The drawing under review shows one solid part. Ordinate dimensions are in mm from its lowest x, y, z. Coordinates: 2 decimals unless noted, no trailing zeros. Loops run counter-clockwise (first coordinate to the right, second up) from the corner with the lowest first, then second, coordinate; pieces in that order, holes last. Notation, with made-up numbers: M 64.5,25.25 L 96.5,25.25 A8 cw 96.5,31.25 Z; hole C 25.25,12.25 d11. An arc over 180 degrees is marked long. Answer as a JSON object with one key per item and string values. Group by question number.
1. To check wall thickness, follow probe 1 along X at (y, z) = (1.85, 7.25); probe 2 along X at (y, z) = (2.4, 1.25); probe 3 along Z at (x, y) = (25, 0.65). State the ranges of each line that lie inside material, in increasing order.
2. Consider section D-D (x = 13). State the section outline as (y, z) points.
3. Consider section C-C (z = 16.5). State the section outline as (x, y) points, then the cut area to 3 significant figures.
4. Consider section A-A (z = 10.25). State the section outline as (x, y) points, then the cut area to 3 significant figures.
5. Consider section B-B (y = 2.1). State the section outline as (x, z) points, then the cut area to 3 significant figures.
6. Insertion check: pin 1 (1.5 mm diameter, centred on y = 0.5, z = 8, fed in from -X); pin 2 (1.5 mm diameter, centred on y = 2.5, z = 15.5, fed in from +X); pin 3 (1.5 mm diameter, centred on x = 23.5, y = 2, fed in from -Z). Each pin has a flat end and moves straight along its axis. Give the tip position at first contact, or say it passes through.
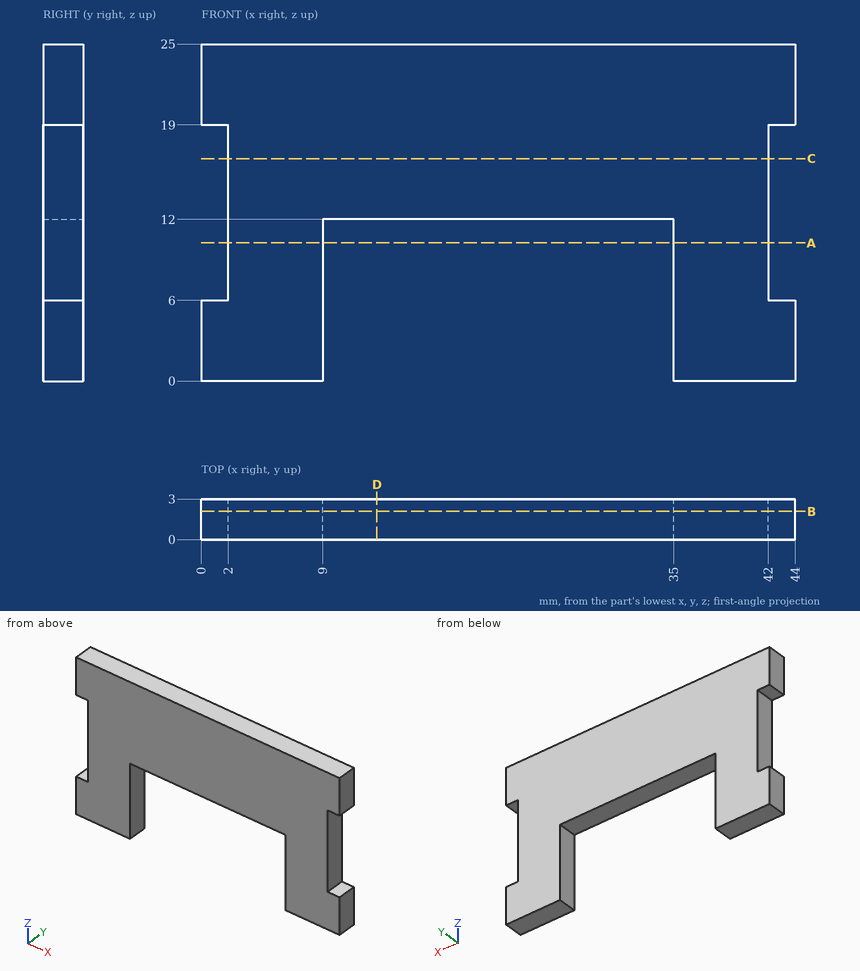
Findings below:
{
 "1": {"probe 1": "x = 2 to 9, 35 to 42", "probe 2": "x = 0 to 9, 35 to 44", "probe 3": "z = 12 to 25"},
 "2": {"outline": "M 0,12 L 3,12 L 3,25 L 0,25 Z"},
 "3": {"outline": "M 2,0 L 42,0 L 42,3 L 2,3 Z", "area": "120 mm^2"},
 "4": {"outline": "M 2,0 L 9,0 L 9,3 L 2,3 Z; M 35,0 L 42,0 L 42,3 L 35,3 Z", "area": "42.0 mm^2"},
 "5": {"outline": "M 0,0 L 9,0 L 9,12 L 35,12 L 35,0 L 44,0 L 44,6 L 42,6 L 42,19 L 44,19 L 44,25 L 0,25 L 0,19 L 2,19 L 2,6 L 0,6 Z", "area": "736 mm^2"},
 "6": {"pin 1": "stops at x = 2", "pin 2": "stops at x = 42", "pin 3": "stops at z = 12"}
}
